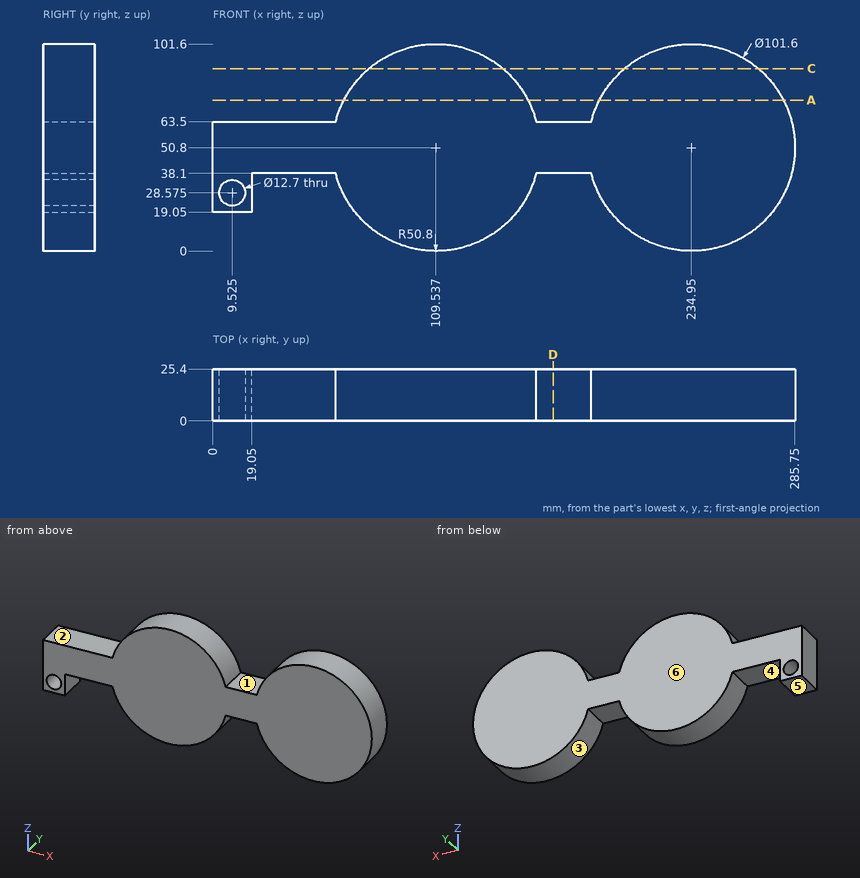
Answer from the drawing. Dimensions are ordinates in mm from the lowest x, y and z of the part. A direction names the side the tool comes from. Give positions to 0.01 mm unless a question says otherwise; leave off trailing zeros. Write each loop counter-clockwise with the first axis right and the second up, starting at its lowest first coordinate (ties: lowest second). Pieces come first, ordered by that corner, then holes. Notation, with made-up numbers: M 4,33.25 L 8,33.25 A17 cw 8,64.25 Z; hole C -34,76 d5. An arc over 180 degrees is marked long. Answer as CSV lines item,"result".
Q1. A cutting plane is placed at C-C on z = 89.5. Write down the section's boundary in (x, y) (1 decimal).
A:
outline,"M 76.6,0 L 142.4,0 L 142.4,25.4 L 76.6,25.4 Z; M 202,0 L 267.9,0 L 267.9,25.4 L 202,25.4 Z"
Q2. A cutting plane is placed at A-A on z = 74. Write down the section's boundary in (x, y) (1 decimal).
A:
outline,"M 64.3,0 L 154.7,0 L 154.7,25.4 L 64.3,25.4 Z; M 189.8,0 L 280.1,0 L 280.1,25.4 L 189.8,25.4 Z"
Q3. Find the intervals of material crossed by probe 1 along Z at (x, y) = (161, 15.5); probe 2 along X at (y, z) = (19.5, 68); probe 3 along X at (y, z) = (3.25, 69) (1 decimal), in increasing order. Write a range as [from, to].
A:
probe 1,"z = [38.1, 63.5]"
probe 2,"x = [61.74, 157.34], [187.15, 282.75]"
probe 3,"x = [62.1, 157], [187.5, 282.4]"
Q4. The mould has two halves that part along X. Classify the marked faces 1, 2 and 3: +X half, -X half, draft (parallel to the pull), parting line (faces both ways), or undercut.
A:
face 1,"undercut"
face 2,"draft"
face 3,"undercut"
Q5. A cutting plane is placed at D-D on x = 167. Write down the section's boundary in (y, z), plus the area to 3 significant figures.
A:
outline,"M 0,38.1 L 25.4,38.1 L 25.4,63.5 L 0,63.5 Z"
area,"645 mm²"
Q6. A tool of negligible diameter and unlimited length cuts with its end or side. For the marked faces 4, 5 and 6, from which of +Z, -Z, +X, -X, +Y, -Y can it reach the whole face along a straight path? Write none if from no direction.
A:
face 4,"-Z, +Y, -Y"
face 5,"-Z, -X, +Y, -Y"
face 6,"+Z, -Z, +X, -X, +Y"
Q7. Given P1, Ø8, axis at y = 12.5, z = 51.5, coming from the +X side; P2, Ø5.5, axis at y = 18, z = 26.5, coming from the +X side; P3, Ø4, axis at x = 164, y = 10.5, coming from the +Z side, each flat-ended and moving along its own axis, determine where each tip first touches the part or whether it passes through.
A:
P1,"stops at x = 285.75"
P2,"stops at x = 280.95"
P3,"stops at z = 63.5"
